The listing builds one solid part. Answer for the finished solid, in the listing's coordinates (mm). Round coordinates to 2 decimals unless told otherwise and drop trailing zeros. Order: outer loops, then holes, each group sorted by start corner. A loop starts at its lowest first (then second) coordinate and runs counter-clockwise, first axis right, second up. Notation, with made-up numbers: M -31,82 L 7,82 A22 cw 7,121 Z; hole C -6,-2 d6. An arc over 180 degrees is marked long. Write item = value, one per line. Start each with the question number.
(1) A cutting plane is placed at B-B, the plane y = -20. Determine the outline of the cut face in (x, z) (3 decimals).
(2) A cutting plane is placed at A-A, the plane x = -1.5. Determine the outline of the cut face in (y, z), and give its area (3 significant figures).
(3) This flat-tipped pin is pushed along its axis until it touches: pin 1 (1 mm diameter, centred on x = -2.5, z = -1.5, fed in from +Y). Where does it stop, or does it pass through?
(4) A cutting plane is placed at C-C, the plane x = 2.5. Determine the outline of the cut face in (y, z).
(5) Straight lines are drawn through the part: probe 1 along Y at (x, z) = (0, -7); probe 2 along Y at (x, z) = (2, 1); probe 3 along Z at (x, y) = (-0.5, -11.75). For each, find the intervals that lie inside material, in ascending order. Write a range as from..to.
(6) A cutting plane is placed at D-D, the plane y = -16.5. Determine the outline of the cut face in (x, z) (3 decimals), and give its area (3 significant figures).
Solid Edge part; units mm, degrees
sketch "Sketch1" plane through (0, 0, 0) normal (1, 0, 0) x (0, 1, 0)
  line L0 (-22.0921, 5.0691) -> (-22.0921, -5.3577)
  arc A0 (-22.0921, -5.3577) -> (-20.7015, -6.7483) centre (-20.7015, -5.3577) ccw
  line L1 (-20.7015, -6.7483) -> (-11.5447, -6.7483)
  arc A1 (-10.1541, -5.3577) -> (-11.5447, -6.7483) centre (-11.5447, -5.3577) cw
  line L2 (-10.1541, -5.3577) -> (-10.1541, 5.0691)
  arc A2 (-11.6065, 6.4583) -> (-10.1541, 5.0691) centre (-11.5447, 5.0691) cw
  arc A3 (-20.6397, 6.4583) -> (-22.0921, 5.0691) centre (-20.7015, 5.0691) ccw
  arc A4 (-11.6065, 6.4583) -> (-20.6397, 6.4583) centre (-16.1231, 107.9579) cw
extrude "Protrusion1" add sketch "Sketch1" along normal mid plane 6.35
fillet "Round_1" radius 1.27 4 edges at (3.175, -22.0921, -0.1443) (-3.175, -22.0921, -0.1443) (3.175, -10.1541, -0.1443) (-3.175, -10.1541, -0.1443)
sketch "Sketch2" plane through (0, -11.6781, -6.7483) normal (0, 0, -1) x (-1, 0, 0)
  circle A0 centre (0, -1.4732) radius 0.4064
  circle A1 centre (0, -7.4168) radius 0.4064
extrude "ExtrudedProtrusion_2" add sketch "Sketch2" along normal blind 2.54
Reported:
q1.outline = M -3.175,-6.748 L 3.175,-6.748 L 3.175,6.432 L -3.175,6.432 Z
q2.outline = M -22.09,-5.36 A1.39 ccw -20.7,-6.75 L -11.54,-6.75 A1.39 ccw -10.15,-5.36 L -10.15,5.07 A1.39 ccw -11.61,6.46 A101.6 cw -20.64,6.46 A1.39 ccw -22.09,5.07 Z
q2.area = 155 mm²
q3.pin_1 = -10.16
q4.outline = M -21.94,-5.98 A1.39 ccw -20.7,-6.75 L -11.54,-6.75 A1.39 ccw -10.3,-5.98 L -10.3,5.69 A1.39 ccw -11.61,6.46 A101.6 cw -20.64,6.46 A1.39 ccw -21.94,5.69 Z
q5.probe_1 = -19.5..-18.69, -13.56..-12.74
q5.probe_2 = -22.09..-10.16
q5.probe_3 = -6.75..6.45
q6.outline = M -3.175,-6.748 L 3.175,-6.748 L 3.175,6.359 L -3.175,6.359 Z
q6.area = 83.2 mm²
